Can you work these out from the drawing? Everything is in mm from the part's minimum corner. A direction names the side the tool comes from. Give positions to 0.01 mm unless a question says otherwise; leave off trailing zeros. Write each loop counter-clockwise with the first axis right and the second up, starting at its lowest first coordinate (ties: lowest second). Pieces come first, ordered by that corner, then holes. Notation, with made-up numbers: (-8.75, 37) - (9.25, 37) arc R5 ccw to (9.25, 41) - close; hole circle Ø1 at (0, 16.25). An arc over 180 degrees is marked (long way). Answer in a Markdown table with one row per item.
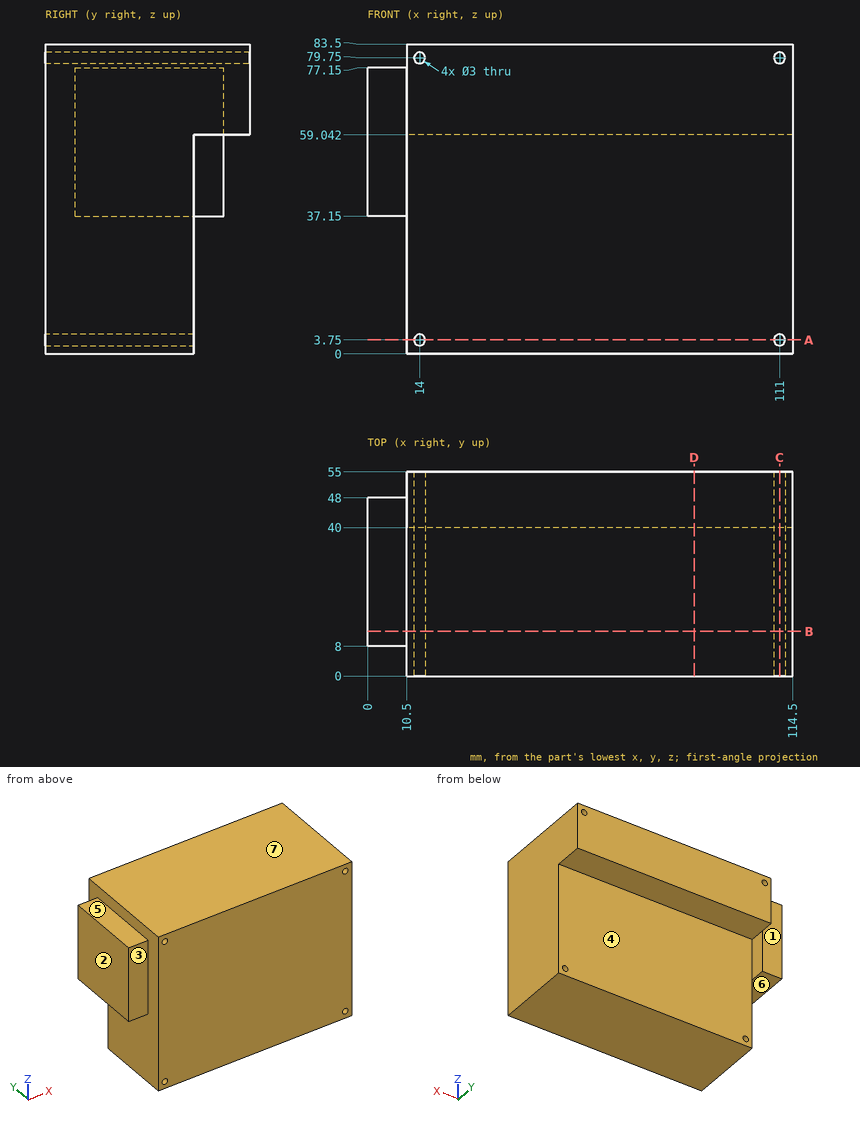
1) On a 3-axis mill with a long thin cutter (end or side, diameter ignored), from which of +Z, -Z, +X, -X, +Y, -Y can I reach the whole of each face in a straight line? I mean the marked faces 4, 5, 6 and 7. Say none if no direction works.
Check values:
| item | result |
|---|---|
| face 4 | -Z, +X, +Y |
| face 5 | +Z, -X, +Y, -Y |
| face 6 | -Z, -X, +Y, -Y |
| face 7 | +Z, +X, -X, +Y, -Y |
2) Will these pins go through, and if not, where does the flat tip stop? P1, Ø5, axis at x = 5.5, y = 37.5, coming from the -Z side; P2, Ø2.5, axis at y = 43, z = 47, coming from the +X side; P3, Ø4.5, axis at x = 65, y = 45, coming from the -Z side; P4, Ø4, axis at y = 46, z = 34.5, coming from the +X side.
Check values:
| item | result |
|---|---|
| P1 | stops at z = 37.15 |
| P2 | stops at x = 10.5 |
| P3 | stops at z = 59.04 |
| P4 | passes through |
3) Imagine slicing it at B-B (y = 12). List the corners of the cut face in (x, z) for me.
Check values:
| item | result |
|---|---|
| outline | (0, 37.15) - (10.5, 37.15) - (10.5, 0) - (114.5, 0) - (114.5, 83.5) - (10.5, 83.5) - (10.5, 77.15) - (0, 77.15) - close; hole circle Ø3 at (14, 3.75); hole circle Ø3 at (14, 79.75); hole circle Ø3 at (111, 3.75); hole circle Ø3 at (111, 79.75) |
4) Imagine slicing it at C-C (x = 111). List the corners of the cut face in (y, z) for me, then the cut area to 3 significant figures.
Check values:
| item | result |
|---|---|
| outline | (0, 0) - (40, 0) - (40, 2.25) - (0, 2.25) - close; (0, 5.25) - (40, 5.25) - (40, 59.04) - (55, 59.04) - (55, 78.25) - (0, 78.25) - close; (0, 81.25) - (55, 81.25) - (55, 83.5) - (0, 83.5) - close |
| area | 3,420 mm2 |
5) Imagine slicing it at A-A (z = 3.75). List the corners of the cut face in (x, y) for me, then the cut area to 3 significant figures.
Check values:
| item | result |
|---|---|
| outline | (10.5, 0) - (12.5, 0) - (12.5, 40) - (10.5, 40) - close; (15.5, 0) - (109.5, 0) - (109.5, 40) - (15.5, 40) - close; (112.5, 0) - (114.5, 0) - (114.5, 40) - (112.5, 40) - close |
| area | 3,920 mm2 |
6) We'd pull the mould along Y, two halves only. Please class the marked faces 1, 2 and 3: +Y half, -Y half, draft (parallel to the pull), parting line (faces both ways), or undercut.
Check values:
| item | result |
|---|---|
| face 1 | +Y half |
| face 2 | draft |
| face 3 | -Y half |
7) Imagine slicing it at D-D (x = 88). List the corners of the cut face in (y, z) for me.
Check values:
| item | result |
|---|---|
| outline | (0, 0) - (40, 0) - (40, 59.04) - (55, 59.04) - (55, 83.5) - (0, 83.5) - close |
8) If I drill on line 1 (X direction, y = 31, z = 80); line 2 (Z direction, x = 111, y = 20); line 3 (X direction, y = 24.5, z = 3), over which ranges is the centre line in solid material (lowest first)?
Check values:
| item | result |
|---|---|
| line 1 | x = 10.5 to 12.52, 15.48 to 109.52, 112.48 to 114.5 |
| line 2 | z = 0 to 2.25, 5.25 to 78.25, 81.25 to 83.5 |
| line 3 | x = 10.5 to 12.7, 15.3 to 109.7, 112.3 to 114.5 |
